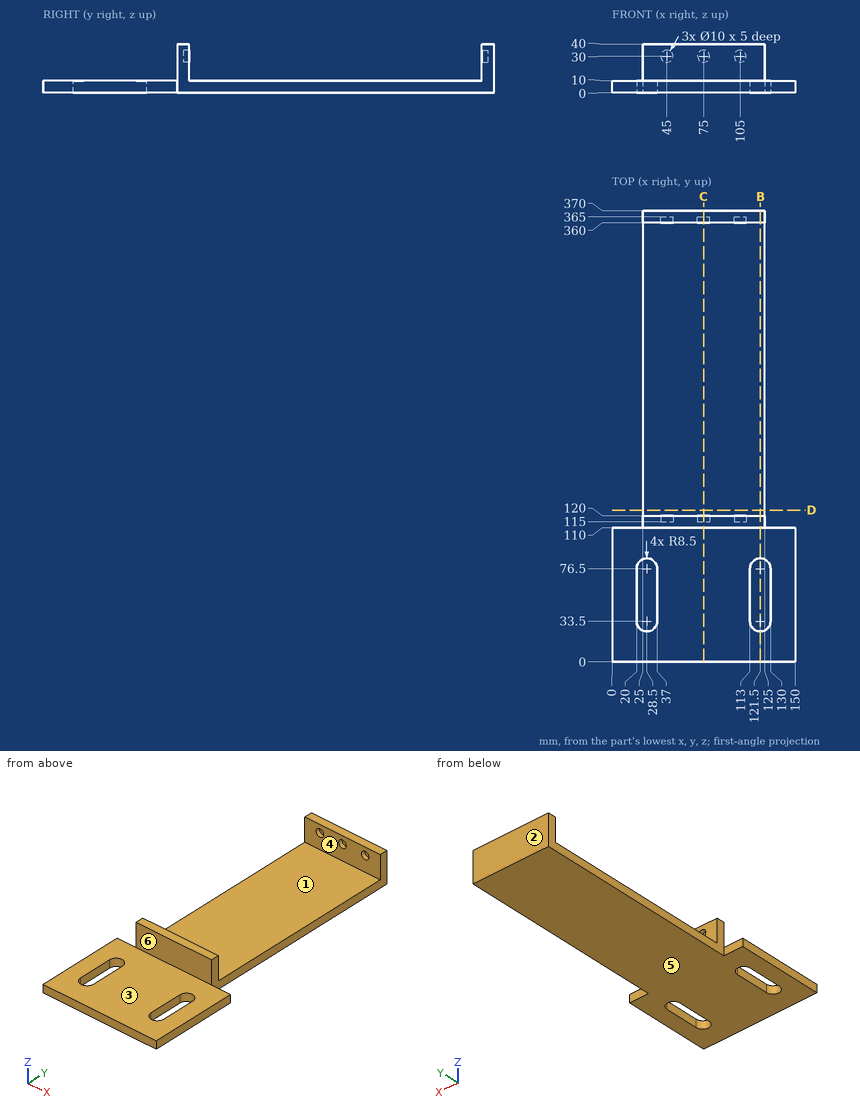
Verification items for this drawing (mm, ordinates from the low corner). A direction names the side the tool comes from. Give positions to 0.01 mm unless a question says otherwise; leave off trailing zeros. Loops run counter-clockwise (first coordinate to the right, second up) from the corner with the lowest first, then second, coordinate; pieces in that order, holes last. Notation, with made-up numbers: M 13.25,9 L 21.25,9 A28 ccw 21.25,40 Z; hole C 9.5,74.5 d2. An arc over 180 degrees is marked long. Return JSON: item names as keys, results as strings. Group by question number.
1. Thickness scan on L1, parallel to X at y = 362, z = 30; L2, parallel to Y at x = 71, z = 22.5; L3, parallel to Z at x = 75, y = 118. Record the ranges inside material, lowest first.
2. Cross-section at C-C on x = 75. Record the boundary of the cut face in (y, z).
3. Go/stop test with flat-tipped pins: pin 1 (12 mm diameter, centred on x = 18, y = 102, fed in from +Z); pin 2 (8 mm diameter, centred on x = 43.5, z = 31.5, fed in from -Y); pin 3 (8 mm diameter, centred on x = 11.5, z = 2.5, fed in from +Y); pin 4 (10 mm diameter, centred on y = 229.5, z = 17, fed in from -X). Record where each tip stops, or that it passes through.
4. Cross-section at B-B on x = 121.5. Record the boundary of the cut face in (y, z), plus the area to 3 significant figures.
5. Cross-section at D-D on y = 124.5. Record the boundary of the cut face in (x, z), plus the area to 3 significant figures.
6. Mould release check, pull along Y, two halves, no side actions. Record for the marked faces 1, 2, 3 and 4: released by +Y, released by -Y, zero draft, split by the parting line, or undercut.
7. Tool access check on the marked faces 5 and 6. Record the directions out of +Z, -Z, +X, -X, +Y, -Y that give a thin tool (end or side, any length) a straight path to the whole face; none if there is none.
Return value:
{
 "1": {"L1": "25 to 40, 50 to 70, 80 to 100, 110 to 125", "L2": "110 to 120, 360 to 370", "L3": "0 to 25, 35 to 40"},
 "2": {"outline": "M 0,0 L 370,0 L 370,40 L 360,40 L 360,35 L 365,35 L 365,25 L 360,25 L 360,10 L 120,10 L 120,25 L 115,25 L 115,35 L 120,35 L 120,40 L 110,40 L 110,10 L 0,10 Z"},
 "3": {"pin 1": "z = 10", "pin 2": "y = 110", "pin 3": "y = 110", "pin 4": "through"},
 "4": {"outline": "M 0,0 L 25,0 L 25,10 L 0,10 Z; M 85,0 L 370,0 L 370,40 L 360,40 L 360,10 L 120,10 L 120,40 L 110,40 L 110,10 L 85,10 Z", "area": "3,700 mm^2"},
 "5": {"outline": "M 25,0 L 125,0 L 125,10 L 25,10 Z", "area": "1,000 mm^2"},
 "6": {"face 1": "undercut", "face 2": "released by +Y", "face 3": "zero draft", "face 4": "undercut"},
 "7": {"face 5": "-Z, +X, -X, +Y, -Y", "face 6": "+Z, +X, -X, -Y"}
}
